Design review of the part built by this model. Coordinates are the model's own, in mm. A direction names the side the tool comes from. Coordinates: 2 decimals unless noted, no trailing zeros. Write each loop counter-clockwise with the first axis right and the second up, starting at its lowest first coordinate (ties: lowest second). Pieces come first, ordered by that corner, then holes. Notation, with made-up numbers: M -15.75,24.5 L 26.25,24.5 A23 ccw 26.25,35.5 Z; hole C -34.75,85 d1. An arc over 180 degrees is marked long. Return JSON: item names as keys, results as strings. Group by question number.
```python
from build123d import *

# Parameters (mm, degrees)
F0_R     = 4.75
F1_DEPTH = 2.45
F2_R     = 3.65
F3_DEPTH = 6.55
F4_W     = 0.6
F4_H     = 2
F5_DEPTH = 5.83
F6_R     = 0.99999


# Not quite as in the source:
# - a fillet or chamfer is up to 0.001 mm smaller than in the source, because OpenCascade refuses the exact size


with BuildPart() as f1:
    # F0 (on Top) → F1 (new body)
    with BuildSketch(Plane.XY):
        Circle(F0_R)
    extrude(amount=-F1_DEPTH)

    # F2 (on face) → F3 (join)
    with BuildSketch(Plane(origin=(0, 0, -2.45), x_dir=(1, 0, 0), z_dir=(0, 0, -1))):
        Circle(F2_R)
    extrude(amount=F3_DEPTH)

    # F4 (on face) → F5 (join)
    with BuildSketch(Plane(origin=(0, 0, -9), x_dir=(1, 0, 0), z_dir=(0, 0, -1))):
        with Locations((-2.05, 0)):
            Rectangle(F4_W, F4_H)
        with Locations((2.05, 0)):
            Rectangle(F4_W, F4_H)
    extrude(amount=F5_DEPTH)

    # F6 (radius 1 in the source; OpenCascade refuses exactly that, so slightly less here)
    f6_edges = [f1.edges().sort_by_distance(p)[0] for p in [
        (-2.05, -1, -14.83),
        (2.05, -1, -14.83),
        (2.05, 1, -14.83),
        (-2.05, 1, -14.83),
    ]]
    fillet(f6_edges, radius=F6_R)


solid = f1.part
```
Item 1: For pin 1 (2 mm diameter, centred on x = 0, y = 3.5, fed in from -Z); pin 2 (2 mm diameter, centred on y = 0, z = -13, fed in from +X); pin 3 (0.5 mm diameter, centred on x = 2, z = -12.5, fed in from +Y), all flat-tipped, find the tip position at first contact; note any pin that passes through.
Item 2: Add section C-C (y = -1.75). Write out the cut boundary in (x, z).
Item 3: Add section B-B (x = 0). Write out the cut boundary in (y, z).
Item 4: For line 1 (X direction, y = 0, z = -6.5); line 2 (X direction, y = -0.75, z = -10); line 3 (Z direction, x = 0, y = 0), list the stretches that pass through material, from the lowest coordinate up.
Item 5: The part is to be moulded in two halves that separate along X. For faces 1 (the flat face through (-1.75, 0, -12)), 2 (the flat face through (-4, 1, -2.45)), 3 (the cylindrical face through (2.192, -4.214, -1.208)), say which applies: pulls with the +X half, pulls with the -X half, needs draft (parallel to the pull), parting line crosses it, or undercut.
Item 6: Add section A-A (z = -9.75). Write out the cut boundary in (x, y), plus the area to 3 significant figures.
Item 7: Machinability: for faces 4 (the flat face through (1.75, 0, -12)), 5 (the flat face through (2.35, 0, -12)), 6 (the flat face through (-2.35, 0, -12)), 7 (the cylindrical face through (3.48, -1.1, -5.68)), which of the approach directions +Z, -Z, +X, -X, +Y, -Y give a long, thin tool a straight path to every point of the face, cutting with its end or side? Answer none if there is none.
Item 8: Add section D-D (z = -1.5). Write out the cut boundary in (x, y).
Geometry check:
{
 "1": {"pin 1": "z = -9", "pin 2": "x = 2.35", "pin 3": "y = 1"},
 "2": {"outline": "M -4.42,-2.45 L -3.2,-2.45 L -3.2,-9 L 3.2,-9 L 3.2,-2.45 L 4.42,-2.45 L 4.42,0 L -4.42,0 Z"},
 "3": {"outline": "M -4.75,-2.45 L -3.65,-2.45 L -3.65,-9 L 3.65,-9 L 3.65,-2.45 L 4.75,-2.45 L 4.75,0 L -4.75,0 Z"},
 "4": {"line 1": "-3.65 to 3.65", "line 2": "-2.35 to -1.75, 1.75 to 2.35", "line 3": "-9 to 0"},
 "5": {"face 1": "undercut", "face 2": "needs draft", "face 3": "parting line crosses it"},
 "6": {"outline": "M -2.35,-1 L -1.75,-1 L -1.75,1 L -2.35,1 Z; M 1.75,-1 L 2.35,-1 L 2.35,1 L 1.75,1 Z", "area": "2.40 mm^2"},
 "7": {"face 4": "-Z, +Y, -Y", "face 5": "-Z, +X, +Y, -Y", "face 6": "-Z, -X, +Y, -Y", "face 7": "-Z"},
 "8": {"outline": "C 0,0 d9.5"}
}
